from build123d import *

# Parameters (mm, degrees)
BOSS_EXTRUDE1_DEPTH   = 50
BOSS_EXTRUDE1_2_DEPTH = 50
BOSS_EXTRUDE2_DEPTH   = 10
CHAMFER1_SIZE         = 15
CHAMFER1_SIZE_2       = 20
SKETCH4_W             = 160
SKETCH4_H             = 200
BOSS_EXTRUDE3_DEPTH   = 5
FILLET1_R             = 10
SKETCH5_R             = 7.5
CUT_EXTRUDE1_DEPTH    = 5
CUT_EXTRUDE3_DEPTH    = 55
FILLET3_R             = 15
FILLET4_R             = 5
SKETCH9_R             = 2
CUT_EXTRUDE4_DEPTH    = 10
FILLET6_R             = 5


with BuildPart() as part:
    # Sketch2 → Boss-Extrude1 (new body)
    with BuildSketch(Plane.XY):
        with BuildLine():
            Line((-50, 75), (-22.70223243, 0))
            Line((-22.70223243, 0), (-37.64392369, -17.092022104))
            ThreePointArc((-37.64392369, -17.092022104), (-49.971924127, -51.675350432), (-35.355339059, -85.355339059))
            Line((-35.355339059, -85.355339059), (-50, -100))
            Line((-50, -100), (-80, -100))
            Line((-80, -100), (-80, 100))
            Line((-80, 100), (-50, 100))
            Line((-50, 100), (-50, 75))
        make_face()
    extrude(amount=-BOSS_EXTRUDE1_DEPTH)



with BuildPart() as body_2:
    # Sketch2 → Boss-Extrude1 2 (new body)
    with BuildSketch(Plane.XY):
        with BuildLine():
            Line((50, 75), (22.70223243, 0))
            Line((22.70223243, 0), (37.64392369, -17.092022104))
            ThreePointArc((37.64392369, -17.092022104), (49.971924127, -51.675350432), (35.355339059, -85.355339059))
            Line((35.355339059, -85.355339059), (50, -100))
            Line((50, -100), (80, -100))
            Line((80, -100), (80, 100))
            Line((80, 100), (50, 100))
            Line((50, 100), (50, 75))
        make_face()
    extrude(amount=-BOSS_EXTRUDE1_2_DEPTH)


with BuildPart() as part_1:
    add(part.part)

    add(body_2.part)  # Boss-Extrude2 merges body 2
    # Sketch3 → Boss-Extrude2 (add)
    with BuildSketch(Plane.XY):
        Polygon((-29.981637115, 20), (29.981637115, 20), (22.70223243, 0), (-22.70223243, 0), align=None)
    extrude(amount=-BOSS_EXTRUDE2_DEPTH)

    # Chamfer1
    # the kernel refuses this chamfer: 20, 15 mm, written as the material it takes off along each edge
    with BuildSketch(Plane(origin=(-81.595588718, 20, -10), x_dir=(0, 0.041308380137954244, 0.9991464445867674), z_dir=(1, 0, 0))) as chamfer1_piece_1_section:
        Polygon((CHAMFER1_SIZE * 0.999146444587, CHAMFER1_SIZE * 0.041308380138), (-CHAMFER1_SIZE_2 * 0.041308380138, CHAMFER1_SIZE_2 * 0.999146444587), (0, 0), align=None)
    chamfer1_piece_1 = extrude(amount=163.191177435, mode=Mode.PRIVATE)
    chamfer1_piece_1 = split(chamfer1_piece_1, bisect_by=Plane(origin=(-24.447399798, 4.794807938, -4.975922198), z_dir=(0.9396926207859094, 0.3420201433256661, 0)), keep=Keep.TOP, mode=Mode.PRIVATE)
    chamfer1_piece_1 = split(chamfer1_piece_1, bisect_by=Plane(origin=(24.447399798, 4.794807938, -4.975922198), z_dir=(-0.939692620785907, 0.34202014332567265, 0)), keep=Keep.TOP, mode=Mode.PRIVATE)
    add(chamfer1_piece_1, mode=Mode.SUBTRACT)

    # Sketch4 → Boss-Extrude3 (add)
    with BuildSketch(Plane.XY):
        Rectangle(SKETCH4_W, SKETCH4_H)
    extrude(amount=BOSS_EXTRUDE3_DEPTH)

    # Fillet1
    fillet1_edges = [part_1.edges().sort_by_distance(p)[0] for p in [
        (0, 13.333333333, 0),
        (-22.70223243, 0, -30),
        (-35.355339059, -85.355339059, -25),
        (35.355339059, -85.355339059, -25),
        (22.70223243, 0, -30),
    ]]
    fillet(fillet1_edges, radius=FILLET1_R)

    # Sketch5 → Cut-Extrude1 (cut)
    with BuildSketch(Plane(origin=(0, 0, 0), x_dir=(-1, 0, 0), z_dir=(0, 0, -1))):
        with Locations((0, -50)):
            Circle(SKETCH5_R)
    extrude(amount=-CUT_EXTRUDE1_DEPTH, mode=Mode.SUBTRACT)

    # Sketch8 → Cut-Extrude3 (cut)
    with BuildSketch(Plane(origin=(0, 0, -50), x_dir=(-1, 0, 0), z_dir=(0, 0, -1))):
        with BuildLine():
            Line((-60, 100), (-80, 100))
            Line((-80, 100), (-80, -100))
            Line((-80, -100), (-58.41745651, -100))
            Line((-58.41745651, -100), (-58.898864587, -85.084522946))
            Line((-58.898864587, -85.084522946), (-59.968772691, -51.935536587))
            ThreePointArc((-59.968772691, -51.935536587), (-56.503917554, -29.818144261), (-45.172708428, -10.510426525))
            Line((-45.172708428, -10.510426525), (-34.120235365, 2.132661237))
            Line((-34.120235365, 2.132661237), (-60, 73.236730193))
            Line((-60, 73.236730193), (-64.733567494, 90.51871221))
            ThreePointArc((-64.733567494, 90.51871221), (-63.462787034, 97.049194521), (-57.5, 100))
            Line((-57.5, 100), (-60, 100))
        make_face()
        with BuildLine():
            Line((34.120235365, 2.132661237), (45.172708428, -10.510426525))
            ThreePointArc((45.172708428, -10.510426525), (56.503917554, -29.818144261), (59.968772691, -51.935536587))
            Line((59.968772691, -51.935536587), (58.898864587, -85.084522946))
            Line((58.898864587, -85.084522946), (58.41745651, -100))
            Line((58.41745651, -100), (80, -100))
            Line((80, -100), (80, 100))
            Line((80, 100), (60, 100))
            Line((60, 100), (57.5, 100))
            ThreePointArc((57.5, 100), (63.462787034, 97.049194521), (64.733567494, 90.51871221))
            Line((64.733567494, 90.51871221), (60, 73.236730193))
            Line((60, 73.236730193), (34.120235365, 2.132661237))
        make_face()
    extrude(amount=-CUT_EXTRUDE3_DEPTH, mode=Mode.SUBTRACT)

    # Fillet3
    fillet3_edges = [part_1.edges().sort_by_distance(p)[0] for p in [
        (34.120235365, 2.132661237, -22.5),
        (-34.120235365, 2.132661237, -22.5),
    ]]
    fillet(fillet3_edges, radius=FILLET3_R)

    # Fillet4
    fillet4_edges = [part_1.edges().sort_by_distance(p)[0] for p in [
        (-50, 100, -25),
        (50, 100, -25),
    ]]
    fillet(fillet4_edges, radius=FILLET4_R)

    # Sketch9 → Cut-Extrude4 (cut)
    with BuildSketch(Plane(origin=(0, 0, -50), x_dir=(-1, 0, 0), z_dir=(0, 0, -1))):
        with Locations((-57.5, 92.5)):
            Circle(SKETCH9_R)
        with Locations((-48.939097244, -85.598196118)):
            Circle(SKETCH9_R)
        with Locations(Location((48.939097244, -85.598196118, 0), (0, 0, 180))):
            Circle(SKETCH9_R)
        with Locations(Location((57.5, 92.5, 0), (0, 0, 180))):
            Circle(SKETCH9_R)
    extrude(amount=-CUT_EXTRUDE4_DEPTH, mode=Mode.SUBTRACT)

    # Fillet6
    fillet6_edges = [part_1.edges().sort_by_distance(p)[0] for p in [
        (58.41745651, -100, -22.5),
        (-58.41745651, -100, -22.5),
    ]]
    fillet(fillet6_edges, radius=FILLET6_R)


solid = part_1.part
Geometry: final body of the model. Coordinates: model frame, mm. A direction names the side the tool comes from. Coordinates: 2 decimals unless noted, no trailing zeros. Loops run counter-clockwise (first coordinate to the right, second up) from the corner with the lowest first, then second, coordinate; pieces in that order, holes last. Notation, with made-up numbers: M 49.25,29.5 L 87.25,29.5 A12 ccw 87.25,47.5 Z; hole C 11.5,80 d8. An arc over 180 degrees is marked long. One line per item, written item: value. Start each with the question number.
1) Cut plane C-C (z = -43). Count the separate pieces of the cut face and the enclosed holes in it, then the cut area to 3 significant figures.
2) Reachability of faces 5 (the flat face through (-48.736, 42.289, -22.885)), 6 (the cylindrical face through (24.277, 0.37, -28.227)), 7 (the flat face through (50, 85, -25)), 8 (the flat face through (62.334, 81.757, -22.885)), 9 (the flat face through (0, 0, -5)) from +Z, -Z, +X, -X, +Y, -Y: full face, straight path, thin tool, end or side. Return the list, or none.
3) Cut plane D-D (y = 69). Return loops of the section in (x, z), then the cut area to 3 significant figures.
4) Cut plane B-B (y = 92.5). Return loops of the section in (x, z), then the cut area to 3 significant figures.
5) Pin query (flat end, axial travel): P1, Ø3, axis at x = -21.5, z = -20.5, coming from the +Y side; P2, Ø1, axis at y = -30.5, z = -8, coming from the +X side; P3, Ø10, axis at y = 83, z = -19.5, coming from the -X side; P4, Ø3.5, axis at x = -57.5, y = 92.5, coming from the -Z side. Return the tip coordinate at first contact, or that it passes through.
6) Material intervals for L1, parallel to Y at x = 0, z = 0.5; L2, parallel to X at y = 91.5, z = -45.5; L3, parallel to X at y = 92, z = -47, sorted ascending. Write a range as from..to.
7) Cut plane A-A (x = 0). Return loops of the section in (y, z), then the cut area to 3 significant figures.
8) Draft query along Y for faces 1 (the flat face through (-1, 68, 0)), 2 (the cylindrical face through (-52, 99, -25)), 3 (the cylindrical face through (-57.76, 90.517, -45.07)), 4 (the flat face through (46, -96, -25)). Return one class per face: released by +Y, released by -Y, zero draft, split by the parting line, or undercut.
Evaluation:
1. separate pieces: 2
1. enclosed holes: 4
1. area: 4,780 mm^2
2. face 5: +Z, -Z, -X
2. face 6: -Z
2. face 7: -Z, +Y
2. face 8: +Z, -Z, +X, -Y
2. face 9: -Z, -Y
3. outline: M -58.46,-50 L -47.82,-50 L -47.82,0 L 47.82,0 L 47.82,-50 L 58.46,-50 L 58.46,5 L -58.46,5 Z
3. area: 1,650 mm^2
4. outline: M -65,-50 L -59.5,-50 L -59.5,-40 L -55.5,-40 L -55.5,-50 L -50,-50 L -50,0 L 50,0 L 50,-50 L 55.5,-50 L 55.5,-40 L 59.5,-40 L 59.5,-50 L 65,-50 L 65,5 L -65,5 Z
4. area: 2,070 mm^2
5. P1: through
5. P2: x = 56.91
5. P3: x = -64.04
5. P4: z = -40
6. L1: -100..-57.5, -42.5..100
6. L2: -64.93..-59.23, -55.77..-50, 50..55.77, 59.23..64.93
6. L3: -64.98..-59.44, -55.56..-50, 50..55.56, 59.44..64.98
7. outline: M -100,0 L -57.5,0 L -57.5,5 L -100,5 Z; M -42.5,0 L 0,0 L 0,-10 L 10.67,-2 A10 cw 16.67,0 L 100,0 L 100,5 L -42.5,5 Z
7. area: 993 mm^2
8. face 1: zero draft
8. face 2: released by +Y
8. face 3: undercut
8. face 4: released by -Y
